The model under review builds one solid part; all positions refer to its coordinate system, in mm. Face numbers are marked on the shaded views. A direction names the side the tool comes from. Coordinates: 2 decimals unless noted, no trailing zeros. Write each loop counter-clockwise with the first axis right and the second up, starting at its lowest first coordinate (ties: lowest second). Pieces come first, ordered by that corner, then holes. Notation, with made-up numbers: M -1,-10.75 L 32,-10.75 A25 cw 32,11.25 Z; hole C 23.5,3 d11. An arc over 180 degrees is marked long. Answer as CSV lines item,"result". Start each with the question number.
from build123d import *

# Parameters (mm, degrees)
F0_W     = 1981.2
F0_H     = 1612.9
F0_W_2   = 355.6
F0_H_2   = 1219.2
F0_R     = 457.2
F1_DEPTH = 101.6
F2_DEPTH = 208.28


# Not quite as in the source:
# - the program builds the solid bodies; features that only make, move or delete a surface that nothing else refers to are left out


with BuildPart() as f1:
    # F0 (on Top) → F1 (new body)
    with BuildSketch(Plane.XY):
        with Locations((-228.6, -50.8)):
            Rectangle(F0_W, F0_H)
        with Locations((-911.225, 114.3)):
            Rectangle(F0_W_2, F0_H_2, mode=Mode.SUBTRACT)
        with Locations((-214.3125, 0)):
            Circle(F0_R, mode=Mode.SUBTRACT)
        with Locations((482.6, 114.3)):
            Rectangle(F0_W_2, F0_H_2, mode=Mode.SUBTRACT)
    extrude(amount=F1_DEPTH)

    # F2 (add): a face of the model
    f2_faces = [f1.faces().sort_by_distance(p)[0] for p in [
        (736.4527890955, -50.8, 101.6),
    ]]
    extrude(f2_faces, amount=F2_DEPTH)


solid = f1.part
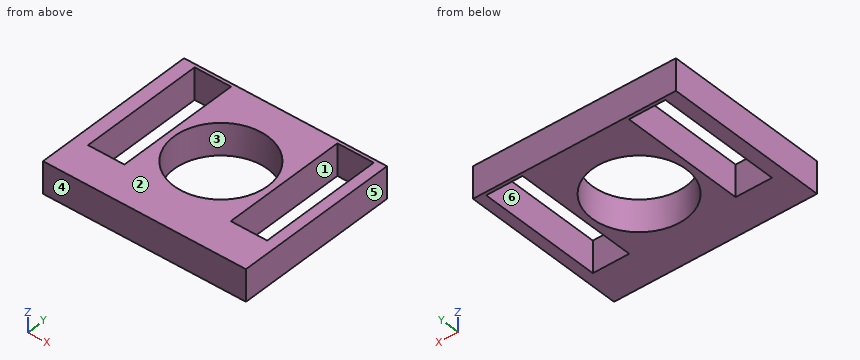
1) Mouldability with a two-part tool opening along X and no side actions: class the marked faces 3, 4, 5 and 6 as +X half, -X half, draft (parallel to the pull), parting line (faces both ways), or undercut.
2) Take a section at D-D on z = 101. Give the number of separate pieces and of enclosed holes in the cut face, and give its area (3 significant figures).
3) To check wall thickness, follow line 1 (Y direction, x = -763, z = 188); line 2 (X direction, y = 320.5, z = 60.5) (3 decimals); line 3 (X direction, y = -414, z = 214) (3 decimals). State the ranges of each line that lie inside material, in increasing order. Write a range as [from, to].
4) Tool access review of the marked faces 1 and 2: name each direction out of +Z, -Z, +X, -X, +Y, -Y from which nothing blocks a thin tool from reaching the whole face with its end or side.
5) Take a section at A-A on y = 0. Give the boundary of the cut face in (x, z) (1 decimal).
6) Take a section at C-C on y = 516.5. Give the boundary of the cut face in (x, z) (3 decimals).
7) Take a section at B-B on x = 548. Give the boundary of the cut face in (y, z).
Results:
1,face 3,"undercut"
1,face 4,"draft"
1,face 5,"+X half"
1,face 6,"undercut"
2,separate pieces,"1"
2,enclosed holes,"3"
2,area,"1,670,000 mm²"
3,line 1,"y = [-857.25, -495.3], [723.9, 755.65]"
3,line 2,"x = [-1219.2, -1089.025], [-733.425, -540.367], [111.742, 304.8], [660.4, 762]"
3,line 3,"x = [-1219.2, -1089.025], [-733.425, -408.312], [-20.313, 304.8], [660.4, 762]"
4,face 1,"+Z, -Z"
4,face 2,"+Z, +X, -X, +Y, -Y"
5,outline,"M -1219.2,0 L -1089,0 L -1089,309.9 L -1219.2,309.9 Z; M -733.4,0 L -671.5,0 L -671.5,309.9 L -733.4,309.9 Z; M 242.9,0 L 304.8,0 L 304.8,309.9 L 242.9,309.9 Z; M 660.4,0 L 762,0 L 762,309.9 L 660.4,309.9 Z"
6,outline,"M -1219.2,0 L -1089.025,0 L -1089.025,309.88 L -1219.2,309.88 Z; M -733.425,0 L 304.8,0 L 304.8,309.88 L -733.425,309.88 Z; M 660.4,0 L 762,0 L 762,309.88 L 660.4,309.88 Z"
7,outline,"M -857.25,0 L -495.3,0 L -495.3,309.88 L -857.25,309.88 Z; M 723.9,0 L 755.65,0 L 755.65,309.88 L 723.9,309.88 Z"
